Could you check a few things on this model? Use its own coordinates, in mm. Face numbers are marked on the shaded views. A direction names the side the tool comes from. Give positions to 0.01 mm unless a question says otherwise; leave off trailing zeros. Loops run counter-clockwise (first coordinate to the right, second up) from the corner with the lowest first, then second, coordinate; pieces in that order, holes last. Notation, with made-up numbers: M 73.25,-2.5 L 98.25,-2.5 A20 ccw 98.25,20.5 Z; hole C 36.25,69 d11. An arc over 180 degrees is marked long. Use a Markdown table: item, result. Add a question column.
1) Suppose I cut it at A-A on x = 0. List the corners of the cut face in (y, z) for me.
2) Suppose I cut it at B-B on x = -47.5. List the corners of the cut face in (y, z) for me.
3) Suppose I cut it at C-C on y = 3. List the corners of the cut face in (x, z) for me.
4) We'd pull the mould along X, two halves only. Please class the marked faces 3, 4 and 5: +X half, -X half, draft (parallel to the pull), parting line (faces both ways), or undercut.
5) Will these pins go through, and if not, where does the flat tip stop? pin 1 Ø4 at (x, z) = (-15.5, 5.5) entering from +Y; pin 2 Ø2 at (y, z) = (9.5, 1) entering from +X; pin 3 Ø2.5 at (x, z) = (-2.5, 4.5) entering from -Y.
6) Which directions (+Z, -Z, +X, -X, +Y, -Y) give clear straight access to the entire face, cutting with the end or side of a thin tool? Please do the marked faces 1 and 2.
7) If I drill on line 1 along Y through (x, z) = (47.5, 5.5); line 2 along X through (y, z) = (6.5, 4.5); line 3 along Y through (x, z) = (-17.5, 3), over which ranges is the centre line in solid material (lowest first)? Write a range as [from, to].
8) Suppose I cut it at D-D on z = 3.5. List the corners of the cut face in (x, y) for me, and give its area (3 significant figures).
```python
from build123d import *

# Parameters (mm, degrees)
SKETCH1_R           = 4.5
BOSS_EXTRUDE1_DEPTH = 8


with BuildPart() as part:
    # Sketch1 → Boss-Extrude1 (new body)
    with BuildSketch(Plane.XY):
        with BuildLine():
            Line((45.179528047, 16.128442524), (7.43557573, -15.258633613))
            ThreePointArc((7.43557573, -15.258633613), (-0.001652224, -23.739558281), (-7.43514282, -15.255357644))
            Line((-7.43514282, -15.255357644), (-45.17916835, 16.128559565))
            ThreePointArc((-45.17916835, 16.128559565), (-54.553423072, 25.809798901), (-41.15571123, 27.260441537))
            Line((-41.15571123, 27.260441537), (41.15571123, 27.260441537))
            ThreePointArc((41.15571123, 27.260441537), (54.553358782, 25.809976769), (45.179528047, 16.128442524))
        make_face()
        with Locations((-47.5, 23.260441537)):
            Circle(SKETCH1_R, mode=Mode.SUBTRACT)
        with Locations((47.5, 23.260441537)):
            Circle(SKETCH1_R, mode=Mode.SUBTRACT)
        with Locations((0, -16.239558463)):
            Circle(SKETCH1_R, mode=Mode.SUBTRACT)
        with BuildLine():
            Line((36.433890862, 19.260441537), (2.320471953, -9.107559451))
            ThreePointArc((2.320471953, -9.107559451), (-0.001660699, -8.739558647), (-2.323630152, -9.108587778))
            Line((-2.323630152, -9.108587778), (-36.434768163, 19.260441537))
            Line((-36.434768163, 19.260441537), (36.433890862, 19.260441537))
        make_face(mode=Mode.SUBTRACT)
    extrude(amount=BOSS_EXTRUDE1_DEPTH)


solid = part.part
```
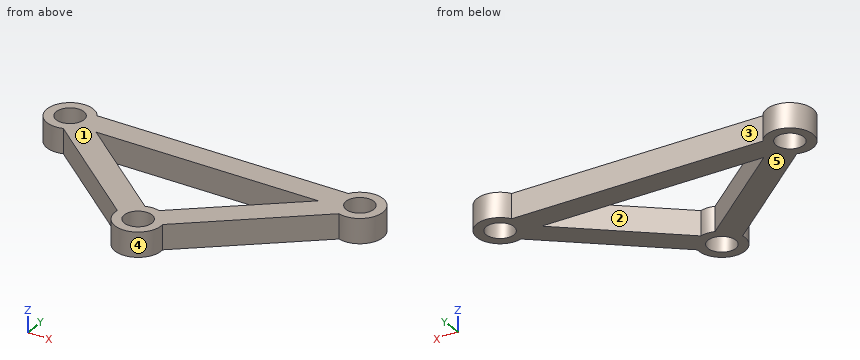
Answer block:
| question | item | result |
|---|---|---|
| 1 | outline | M -23.74,0 L -20.74,0 L -20.74,8 L -23.74,8 Z; M -11.74,0 L -8.74,0 L -8.74,8 L -11.74,8 Z; M 19.26,0 L 27.26,0 L 27.26,8 L 19.26,8 Z |
| 2 | outline | M 15.76,0 L 18.76,0 L 18.76,8 L 15.76,8 Z; M 27.76,0 L 30.76,0 L 30.76,8 L 27.76,8 Z |
| 3 | outline | M -29.39,0 L -16.88,0 L -16.88,8 L -29.39,8 Z; M 16.88,0 L 29.39,0 L 29.39,8 L 16.88,8 Z |
| 4 | face 3 | undercut |
| 4 | face 4 | parting line |
| 4 | face 5 | draft |
| 5 | pin 1 | stops at y = 27.26 |
| 5 | pin 2 | stops at x = 38.41 |
| 5 | pin 3 | stops at y = -23.63 |
| 6 | face 1 | +Z, +X, -X, +Y, -Y |
| 6 | face 2 | +Z, -Z |
| 7 | line 1 | y = [15.76, 18.76], [27.76, 30.76] |
| 7 | line 2 | x = [-33.6, -21.09], [21.09, 33.6] |
| 7 | line 3 | y = [-6.89, 3.51], [19.26, 27.26] |
| 8 | outline | M -45.18,16.13 L -7.44,-15.26 A7.5 ccw long 7.44,-15.26 L 45.18,16.13 A7.5 ccw long 41.16,27.26 L -41.16,27.26 A7.5 ccw long Z; hole C -47.5,23.26 d9; hole M -36.43,19.26 L -2.32,-9.11 A7.5 cw 2.32,-9.11 L 36.43,19.26 Z; hole C 0,-16.24 d9; hole C 47.5,23.26 d9 |
| 8 | area | 1,730 mm^2 |
